Source: CAD feature listing. Evaluate the final solid. Frame: model axes, mm. Face numbers are marked on the shaded views. A direction names the side the tool comes from. Give positions to 0.01 mm unless a question says otherwise; leave off trailing zeros. Loops run counter-clockwise (first coordinate to the right, second up) from the corner with the lowest first, then second, coordinate; pieces in that order, holes last.
```python
from build123d import *

# Parameters (mm, degrees)
SALIENTE_EXTRUIR1_DEPTH = 8
CROQUIS3_W              = 21
CROQUIS3_H              = 15
SALIENTE_EXTRUIR2_DEPTH = 1.5
CROQUIS4_R              = 3
CORTAR_EXTRUIR1_DEPTH   = 9.413938048
CROQUIS5_W              = 12
CROQUIS5_H              = 15
SALIENTE_EXTRUIR3_DEPTH = 7
CORTAR_EXTRUIR2_DEPTH   = 7
REDONDEO1_R             = 1
CHAFL_N1_SIZE           = 0.5
SALIENTE_EXTRUIR4_DEPTH = 1.2
CHAFL_N2_SIZE           = 1


with BuildPart() as part:
    # Croquis1 → Saliente-Extruir1 (new body)
    with BuildSketch(Plane.XY):
        with BuildLine():
            Line((1.928362829, 2.298133329), (3.213938048, 3.830222216))
            ThreePointArc((3.213938048, 3.830222216), (-0.868240888, 4.924038765), (-4.330127019, 2.5))
            Line((-4.330127019, 2.5), (-5.2, 2.5))
            Line((-5.2, 2.5), (-5.2, -2.5))
            Line((-5.2, -2.5), (-4.330127019, -2.5))
            ThreePointArc((-4.330127019, -2.5), (-0.868240888, -4.924038765), (3.213938048, -3.830222216))
            Line((3.213938048, -3.830222216), (1.928362829, -2.298133329))
            ThreePointArc((1.928362829, -2.298133329), (-3, 0), (1.928362829, 2.298133329))
        make_face()
    extrude(amount=SALIENTE_EXTRUIR1_DEPTH)

    # Croquis3 → Saliente-Extruir2 (add)
    with BuildSketch(Plane.ZY.offset(5.2)):
        with Locations((10.5, 0)):
            Rectangle(CROQUIS3_W, CROQUIS3_H)
    extrude(amount=-SALIENTE_EXTRUIR2_DEPTH)

    # Croquis4 → Cortar-Extruir1 (cut, through all)
    with BuildSketch(Plane.ZY.offset(5.2)):
        with Locations((15, 0)):
            Circle(CROQUIS4_R)
    extrude(amount=-CORTAR_EXTRUIR1_DEPTH, mode=Mode.SUBTRACT)

    # Croquis5 → Saliente-Extruir3 (add)
    with BuildSketch(Plane(origin=(-3.7, 0, 0), x_dir=(0, 0, -1), z_dir=(1, 0, 0))):
        with Locations((-15, 0)):
            Rectangle(CROQUIS5_W, CROQUIS5_H)
    extrude(amount=SALIENTE_EXTRUIR3_DEPTH)

    # Croquis7 → Cortar-Extruir2 (cut)
    with BuildSketch(Plane(origin=(3.3, 0, 0), x_dir=(0, 0, -1), z_dir=(1, 0, 0))):
        Polygon((-10, -2.886751346), (-10, 2.886751346), (-15, 5.773502692), (-20, 2.886751346), (-20, -2.886751346), (-15, -5.773502692), align=None)
    extrude(amount=-CORTAR_EXTRUIR2_DEPTH, mode=Mode.SUBTRACT)

    # Redondeo1
    redondeo1_edges = [part.edges().sort_by_distance(p)[0] for p in [
        (1.928362829, -2.298133329, 4),
        (1.928362829, 2.298133329, 4),
    ]]
    fillet(redondeo1_edges, radius=REDONDEO1_R)

    # Chaflán1
    chafl_n1_edges = [part.edges().sort_by_distance(p)[0] for p in [
        (-3, 0, 0),
        (2.851721878, -3.398549793, 0),
        (2.851721878, 3.398549793, 0),
        (1.935447157, 2.632392254, 0),
        (1.935447157, -2.632392254, 0),
    ]]
    chamfer(chafl_n1_edges, length=CHAFL_N1_SIZE)

    # Croquis8 → Saliente-Extruir4 (add)
    with BuildSketch(Plane(origin=(0, 7.5, 0), x_dir=(1, 0, 0), z_dir=(0, 1, 0))):
        Polygon((-3.7, 0), (3.3, -9), (-3.7, -9), align=None)
    saliente_extruir4 = extrude(amount=-SALIENTE_EXTRUIR4_DEPTH)

    # Simetría1: Saliente-Extruir4 across plane
    add(saliente_extruir4.mirror(Plane.ZX))

    # Chaflán2
    chafl_n2_edges = [part.edges().sort_by_distance(p)[0] for p in [
        (-4.45, -7.5, 0),
        (-4.45, 7.5, 0),
        (-0.95, 7.5, 21),
        (-0.95, -7.5, 21),
    ]]
    chamfer(chafl_n2_edges, length=CHAFL_N2_SIZE)


solid = part.part
```
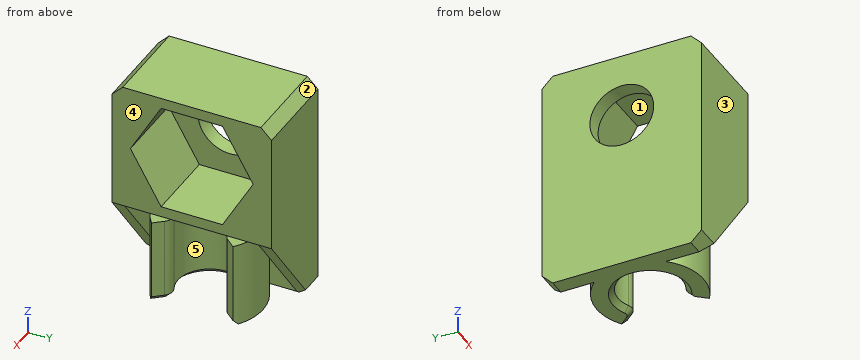
(1) First-contact query: pin 1 (3 mm diameter, centred on y = 2, z = 17, fed in from +X); pin 2 (4.5 mm diameter, centred on y = 1.5, z = 5, fed in from +X); pin 3 (1 mm diameter, centred on x = 2, y = 2.5, fed in from -Z). Flat tips, straight axial feed; report the tip coordinate or a pass-through.
A:
pin 1: stops at x = -3.7
pin 2: stops at x = 3.15
pin 3: stops at z = 0.14
(2) Section A-A, the plane x = 0. Return the cut outline in (y, z), then the cut area to 3 significant figures.
A:
outline: (-7.5, 4.76) - (-6.3, 4.76) - (-6.3, 9) - (6.3, 9) - (6.3, 4.76) - (7.5, 4.76) - (7.5, 20) - (6.5, 21) - (-6.5, 21) - (-7.5, 20) - close; (-5, 0) - (-3.5, 0) - (-3, 0.5) - (-3, 8) - (-5, 8) - close; (3, 0.5) - (3.5, 0) - (5, 0) - (5, 8) - (3, 8) - close; hole (-5.77, 15) - (-2.89, 10) - (2.89, 10) - (5.77, 15) - (2.89, 20) - (-2.89, 20) - close
area: 134 mm2
(3) Ray query, line 1 along Y through (x, z) = (0, 5.75); line 2 along Y through (x, z) = (-1.5, 3.5); line 3 along Y through (x, z) = (0, 4.5). Return the intervals inside material, ascending.
A:
line 1: y = -7.5 to -6.3, -5 to -3, 3 to 5, 6.3 to 7.5
line 2: y = -7.5 to -6.3, -4.77 to -2.6, 2.6 to 4.77, 6.3 to 7.5
line 3: y = -5 to -3, 3 to 5
(4) Reachability of the marked faces 1 and 2 from +Z, -Z, +X, -X, +Y, -Y: full face, straight path, thin tool, end or side. Return the list, or none.
A:
face 1: +X
face 2: +Z, +X, -X, +Y
(5) Section B-B, the plane y = 0. Return the cut outline in (x, z).
A:
outline: (-5.2, 0) - (-3.5, 0) - (-3, 0.5) - (-3, 8) - (-3.7, 8) - (-3.7, 9) - (3.3, 9) - (3.3, 10) - (-3.7, 10) - (-3.7, 12) - (-5.2, 12) - close; (-5.2, 18) - (-3.7, 18) - (-3.7, 20) - (3.3, 20) - (3.3, 21) - (-5.2, 21) - close
(6) Section D-D, the plane x = -1.75. Count the separate pieces of the cut face and the enclosed holes in it, then the cut area to 3 significant figures.
A:
separate pieces: 3
enclosed holes: 1
area: 144 mm2
(7) Section C-C, the plane y = 6. Return the cut outline in (x, z), then the cut area to 4 significant figures.
A:
outline: (-5.2, 0) - (-3.7, 0) - (-3.7, 9) - (3.3, 9) - (3.3, 21) - (-5.2, 21) - close
area: 115.5 mm2
(8) Mould query, pull axis X, two halves, no side actions, for the marked faces 3, 4 and 5. Classes: pulls with the +X half, pulls with the -X half, needs draft (parallel to the pull), parting line crosses it, or undercut.
A:
face 3: needs draft
face 4: pulls with the +X half
face 5: undercut
